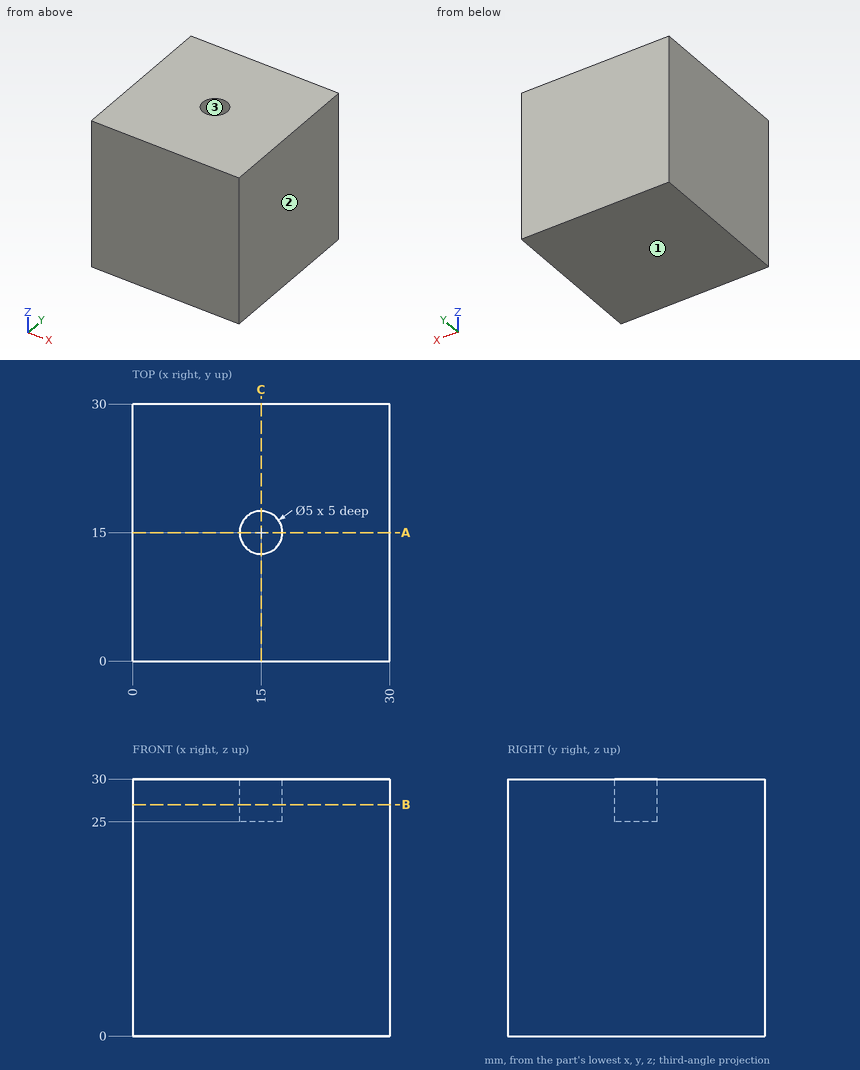
Answer from the drawing. Dimensions are ordinates in mm from the lowest x, y and z of the part. Coordinates: 2 decimals unless noted, no trailing zeros. Loops run counter-clockwise (first coordinate to the right, second up) from the corner with the lowest first, then second, coordinate; pieces in that order, holes last. Notation, with made-up numbers: (-21.5, 25) - (25.5, 25) arc R23 ccw to (25.5, 47) - close; hole circle Ø5 at (52, 8). An arc over 180 degrees is marked (long way). Use a Markdown table: item, result.
Item 1: The mould has two halves that part along X. Classify the marked faces 1, 2 and 3: +X half, -X half, draft (parallel to the pull), parting line (faces both ways), or undercut.
Evaluation:
| item | result |
|---|---|
| face 1 | draft |
| face 2 | +X half |
| face 3 | undercut |
Item 2: Find section B-B, the plane z = 27. Determine the outline of the cut face in (x, y), and give its area (3 significant figures).
Evaluation:
| item | result |
|---|---|
| outline | (0, 0) - (30, 0) - (30, 30) - (0, 30) - close; hole circle Ø5 at (15, 15) |
| area | 880 mm2 |
Item 3: Consider probe 1 along Y at (x, z) = (15, 27.25); probe 2 along Z at (x, y) = (15.5, 14.5). Determine where each line is inside the solid, lowest interval first. Write a range as from..to.
Evaluation:
| item | result |
|---|---|
| probe 1 | y = 0..12.5, 17.5..30 |
| probe 2 | z = 0..25 |
Item 4: Find section A-A, the plane y = 15. Determine the outline of the cut face in (x, z), and give its area (3 significant figures).
Evaluation:
| item | result |
|---|---|
| outline | (0, 0) - (30, 0) - (30, 30) - (17.5, 30) - (17.5, 25) - (12.5, 25) - (12.5, 30) - (0, 30) - close |
| area | 875 mm2 |
